```python
from build123d import *

# Parameters (mm, degrees)
BOSS_EXTRUDE1_DEPTH = 2
BOSS_EXTRUDE2_DEPTH = 5
SKETCH2_R           = 1.4
CUT_EXTRUDE1_DEPTH  = 8
FILLET1_R           = 2


with BuildPart() as part:
    # Sketch1 → Boss-Extrude1 (new body)
    with BuildSketch(Plane.XY):
        Polygon((40.290198527, 15.03487922), (40.290198527, -35.46512078), (44.290198527, -35.46512078), (44.290198527, 19.03487922), (-38.709801473, 19.03487922), (-38.709801473, -35.46512078), (-34.709801473, -35.46512078), (-34.709801473, 15.03487922), align=None)
    extrude(amount=BOSS_EXTRUDE1_DEPTH)

    # Sketch1_4 → Boss-Extrude2 (add)
    with BuildSketch(Plane.XY):
        Polygon((-44.709801473, -35.46512078), (-38.709801473, -35.46512078), (-38.709801473, 19.03487922), (44.290198527, 19.03487922), (44.290198527, -35.46512078), (50.290198527, -35.46512078), (50.290198527, 25.03487922), (5.955198527, 25.03487922), (5.955198527, 29.03487922), (-0.374801473, 29.03487922), (-0.374801473, 25.03487922), (-44.709801473, 25.03487922), align=None)
    extrude(amount=BOSS_EXTRUDE2_DEPTH)

    # Sketch2 → Cut-Extrude1 (cut)
    with BuildSketch(Plane(origin=(5.955198527, 0, 0), x_dir=(0, 0, -1), z_dir=(1, 0, 0))):
        with Locations((-2.5, 27.39487922)):
            Circle(SKETCH2_R)
    extrude(amount=-CUT_EXTRUDE1_DEPTH, mode=Mode.SUBTRACT)

    # Fillet1
    fillet1_edges = [part.edges().sort_by_distance(p)[0] for p in [
        (2.790198527, 29.03487922, 5),
        (2.790198527, 29.03487922, 0),
    ]]
    fillet(fillet1_edges, radius=FILLET1_R)


solid = part.part
```
Model file for the job. Use its own axes, mm. A direction names the side the tool comes from. Round coordinates to 2 decimals unless told otherwise and drop trailing zeros. Loops run counter-clockwise (first coordinate to the right, second up) from the corner with the lowest first, then second, coordinate; pieces in that order, holes last. Notation, with made-up numbers: M 42.25,35 L 75.25,35 A29 ccw 75.25,62 Z; hole C 38,81.5 d11. An arc over 180 degrees is marked long. Put each result on its own line as item: value. Start each with the question number.
Item 1: 3-axis set-ups, long thin cutter, end or side, ignore diameter. For faces 1 (the face through (2, 15.035, 1)), 2 (the face through (5.955, 25.7, 2.5)), 3 (the face through (44.29, -8, 3)), 4 (the face through (-22, 25.035, 2)): which of +Z, -Z, +X, -X, +Y, -Y reach the whole face in a straight line?
Item 2: Drop flat-ended pins along their axis: P1, Ø2, axis at x = 0.5, z = 0.5, coming from the -Y side; P2, Ø6, axis at x = 25, y = 18, coming from the -Z side; P3, Ø2.5, axis at x = 34, z = 2.5, coming from the +Y side; P4, Ø1.5, axis at x = 10.5, z = 3.5, coming from the -Y side. Give the stop position or say it passes through.
Item 3: Mould opens along Y. For faces 5 (the face through (-38.71, -9, 3)), 6 (the face through (2.835, 26.028, 2.803)), 7 (the face through (2, 19.035, 3)) say: released by +Y, released by -Y, zero draft, split by the parting line, or undercut.
Item 4: Drill centre lines: line 1 along Y through (x, z) = (4, 2.5); line 2 along X through (y, z) = (13, 4.7); line 3 along X through (y, z) = (7.5, 1.3). Where is each one in solid material? Low to high.
Item 5: Cut at A-A (y = -4.5). List the corners of the cut face in (x, z), then the cut area to 3 significant figures.
Item 6: Cut at B-B (x = 38). List the corners of the cut face in (y, z), then the cut area to 3 significant figures.
Answer block:
1. face 1: +Z, -Z, -Y
1. face 2: +Z, -Z, +X, +Y
1. face 3: +Z, -Y
1. face 4: +Z, -Z, -X, +Y
2. P1: y = 15.03
2. P2: z = 0
2. P3: y = 25.03
2. P4: y = 19.03
3. face 5: zero draft
3. face 6: undercut
3. face 7: released by -Y
4. line 1: 19.03 to 25.99, 28.79 to 29.03
4. line 2: -44.71 to -38.71, 44.29 to 50.29
4. line 3: -44.71 to -34.71, 40.29 to 50.29
5. outline: M -44.71,0 L -34.71,0 L -34.71,2 L -38.71,2 L -38.71,5 L -44.71,5 Z; M 40.29,0 L 50.29,0 L 50.29,5 L 44.29,5 L 44.29,2 L 40.29,2 Z
5. area: 76.0 mm2
6. outline: M 15.03,0 L 25.03,0 L 25.03,5 L 19.03,5 L 19.03,2 L 15.03,2 Z
6. area: 38.0 mm2
